from build123d import *

# Parameters (mm, degrees)
EXTRUDE_THIN1_DEPTH = 10
SKETCH2_W           = 17.824072676
SKETCH2_H           = 3.5
CUT_EXTRUDE1_DEPTH  = 10
SKETCH3_W           = 9
SKETCH3_H           = 3
BOSS_EXTRUDE1_DEPTH = 10
SKETCH4_R           = 1.75
CUT_EXTRUDE2_DEPTH  = 10
SKETCH5_W           = 15
SKETCH5_H           = 5.349927867
BOSS_EXTRUDE2_DEPTH = 27.0318
SKETCH6_W           = 9
SKETCH6_H           = 3.75
CUT_EXTRUDE3_DEPTH  = 13
BOSS_EXTRUDE3_DEPTH = 15
CUT_EXTRUDE8_REACH  = 67.42
SKETCH8_R           = 1.75
BOSS_EXTRUDE4_DEPTH = 37.0318
CUT_EXTRUDE6_DEPTH  = 11.169767789
SKETCH13_R          = 1.75
CUT_EXTRUDE9_DEPTH  = 3


with BuildPart() as part:
    # Sketch1 → Extrude-Thin1 (new body)
    with BuildSketch(Plane.XY):
        with BuildLine():
            Line((7.5, 8.014450411), (7.5, 13.364378278))
            Line((7.5, 13.364378278), (-7.5, 13.364378278))
            Line((-7.5, 13.364378278), (-7.5, 8.014450411))
            ThreePointArc((-7.5, 8.014450411), (0, -10.556649897), (7.5, 8.014450411))
        make_face()
        with BuildLine():
            Line((4.5, 6.614378278), (4.5, 10.364378278))
            Line((4.5, 10.364378278), (-4.5, 10.364378278))
            Line((-4.5, 10.364378278), (-4.5, 6.614378278))
            ThreePointArc((-4.5, 6.614378278), (0, -7.556649897), (4.5, 6.614378278))
        make_face(mode=Mode.SUBTRACT)
    extrude(amount=-EXTRUDE_THIN1_DEPTH)

    # Sketch2 → Cut-Extrude1 (cut)
    with BuildSketch(Plane(origin=(0, 0, -10), x_dir=(-1, 0, 0), z_dir=(0, 0, -1))):
        with Locations((8.912036338, 0)):
            Rectangle(SKETCH2_W, SKETCH2_H)
    extrude(amount=-CUT_EXTRUDE1_DEPTH, mode=Mode.SUBTRACT)

    # Sketch3 → Boss-Extrude1 (add)
    with BuildSketch(Plane.XY):
        with Locations((-12.153104343, 3.25)):
            Rectangle(SKETCH3_W, SKETCH3_H)
        with Locations((-12.04099167, -3.25)):
            Rectangle(SKETCH3_W, SKETCH3_H)
    extrude(amount=-BOSS_EXTRUDE1_DEPTH)

    # Sketch4 → Cut-Extrude2 (cut)
    with BuildSketch(Plane(origin=(0, 4.75, 0), x_dir=(1, 0, 0), z_dir=(0, 1, 0))):
        with Locations((-13.233947273, 5)):
            Circle(SKETCH4_R)
    extrude(amount=-CUT_EXTRUDE2_DEPTH, mode=Mode.SUBTRACT)

    # Sketch5 → Boss-Extrude2 (add)
    with BuildSketch(Plane.XY):
        with Locations((0, 10.689414345)):
            Rectangle(SKETCH5_W, SKETCH5_H)
    extrude(amount=BOSS_EXTRUDE2_DEPTH)

    # Sketch6 → Cut-Extrude3 (cut)
    with BuildSketch(Plane(origin=(0, 0, -10), x_dir=(-1, 0, 0), z_dir=(0, 0, -1))):
        with Locations((0, 8.489378278)):
            Rectangle(SKETCH6_W, SKETCH6_H)
    extrude(amount=-CUT_EXTRUDE3_DEPTH, mode=Mode.SUBTRACT)

    # Sketch7 → Boss-Extrude3 (add)
    with BuildSketch(Plane.ZY.offset(7.5)):
        Polygon((27.0318, 13.364378278), (-10, 13.364378278), (24.0318, 39.609893084), (24.0318, 51.294233998), (27.0318, 51.294233998), align=None)
    extrude(amount=-BOSS_EXTRUDE3_DEPTH)

    # Cut-Extrude8: up to this face of the body (flat: up to its plane)
    cut_extrude8_end = Plane(part.part.faces().sort_by_distance((0, 29.654342205, 27.0318))[0])
    # Sketch8 → Cut-Extrude8 (cut, up to the picked face)
    with BuildSketch(Plane(origin=(0, 0, -10), x_dir=(-1, 0, 0), z_dir=(0, 0, -1)), mode=Mode.PRIVATE) as cut_extrude8_sk1:
        with Locations(Location((0.697367247, 45.709350103, 0), (0, 0, 90))):
            Circle(SKETCH8_R)
    cut_extrude8_tool1 = split(extrude(cut_extrude8_sk1.sketch, amount=-CUT_EXTRUDE8_REACH, mode=Mode.PRIVATE), bisect_by=cut_extrude8_end, keep=Keep.BOTH, mode=Mode.PRIVATE)
    # Sketch8 → Cut-Extrude8 (cut, up to the picked face)
    with BuildSketch(Plane(origin=(0, 0, -10), x_dir=(-1, 0, 0), z_dir=(0, 0, -1)), mode=Mode.PRIVATE) as cut_extrude8_sk2:
        Polygon((6.282251141, 44.365676022), (6.282251141, 47.053024185), (6.282251141, 51.294233998), (7.5, 51.294233998), (7.5, 39.609893084), (7.5, 13.364378278), align=None)
    cut_extrude8_tool2 = split(extrude(cut_extrude8_sk2.sketch, amount=-CUT_EXTRUDE8_REACH, mode=Mode.PRIVATE), bisect_by=cut_extrude8_end, keep=Keep.BOTH, mode=Mode.PRIVATE)
    # Sketch8 → Cut-Extrude8 (cut, up to the picked face)
    with BuildSketch(Plane(origin=(0, 0, -10), x_dir=(-1, 0, 0), z_dir=(0, 0, -1)), mode=Mode.PRIVATE) as cut_extrude8_sk3:
        Polygon((-4.887516648, 47.053024185), (-4.887516648, 44.365676022), (-7.5, 13.364378278), (-7.5, 39.609893084), (-7.5, 51.294233998), (-4.887516648, 51.294233998), align=None)
    cut_extrude8_tool3 = split(extrude(cut_extrude8_sk3.sketch, amount=-CUT_EXTRUDE8_REACH, mode=Mode.PRIVATE), bisect_by=cut_extrude8_end, keep=Keep.BOTH, mode=Mode.PRIVATE)
    add(cut_extrude8_tool1.solids().sort_by(Axis((-0.697367, 45.70935, -10), (0, 0, 1)))[0], mode=Mode.SUBTRACT)
    add(cut_extrude8_tool2.solids().sort_by(Axis((-7.031388, 38.294234, -10), (0, 0, 1)))[0], mode=Mode.SUBTRACT)
    add(cut_extrude8_tool3.solids().sort_by(Axis((6.494669, 38.294234, -10), (0, 0, 1)))[0], mode=Mode.SUBTRACT)

    # Sketch11 → Boss-Extrude4 (add)
    with BuildSketch(Plane(origin=(0, 0, -10), x_dir=(-1, 0, 0), z_dir=(0, 0, -1))):
        with BuildLine():
            Line((6.282251141, -43.878975815), (6.282251141, -46.566323978))
            Line((6.282251141, -46.566323978), (6.282251141, -50.807533791))
            Line((6.282251141, -50.807533791), (2.041041328, -50.807533791))
            Line((2.041041328, -50.807533791), (-0.646306835, -50.807533791))
            Line((-0.646306835, -50.807533791), (-4.887516648, -50.807533791))
            Line((-4.887516648, -50.807533791), (-4.887516648, -46.566323978))
            Line((-4.887516648, -46.566323978), (-4.887516648, -43.878975815))
            Line((-4.887516648, -43.878975815), (-4.887516648, -5.83548046))
            ThreePointArc((-4.887516648, -5.83548046), (1.037871953, -7.540787293), (6.282251141, -4.298135849))
            Line((6.282251141, -4.298135849), (6.282251141, -43.878975815))
        make_face()
    extrude(amount=-BOSS_EXTRUDE4_DEPTH)

    # Sketch12 → Cut-Extrude6 (cut)
    with BuildSketch(Plane(origin=(-6.282251141, 0, 0), x_dir=(0, 0, -1), z_dir=(1, 0, 0))):
        Polygon((10, -12.309364669), (10, -50.807533791), (-24.0318, -50.807533791), (-24.0318, -39.062586463), align=None)
    extrude(amount=CUT_EXTRUDE6_DEPTH, mode=Mode.SUBTRACT)

    # Sketch13 → Cut-Extrude9 (cut)
    with BuildSketch(Plane.XY.offset(27.0318)):
        with Locations((-0.697367247, -45.222649897)):
            Circle(SKETCH13_R)
    extrude(amount=-CUT_EXTRUDE9_DEPTH, mode=Mode.SUBTRACT)


solid = part.part
Here's how the part is built. I have some questions about the finished solid (model axes, mm). A direction names the side the tool comes from. Coordinates: 2 decimals unless noted, no trailing zeros. Order: outer loops, then holes, each group sorted by start corner. A loop starts at its lowest first (then second) coordinate and runs counter-clockwise, first axis right, second up. Notation, with made-up numbers: M 5,22.5 L 40,22.5 A19 ccw 40,32.5 Z; hole C 84.5,32.5 d2. An arc over 180 degrees is marked long. Answer as CSV lines item,"result".
Item 1: Imagine slicing it at B-B on x = -13.75. Write out the boundary of the cut face in (y, z).
Results found:
outline,"M -4.75,-10 L -1.75,-10 L -1.75,-6.67 L -4.75,-6.67 Z; M -4.75,-3.33 L -1.75,-3.33 L -1.75,0 L -4.75,0 Z; M 1.75,-10 L 4.75,-10 L 4.75,-6.67 L 1.75,-6.67 Z; M 1.75,-3.33 L 4.75,-3.33 L 4.75,0 L 1.75,0 Z"
Item 2: Imagine slicing it at A-A on z = 2. Write out the boundary of the cut face in (x, y), plus the area to 3 significant figures.
Results found:
outline,"M -7.5,8.01 L -4.5,8.01 L -4.5,10.36 L 4.5,10.36 L 4.5,8.01 L 7.5,8.01 L 7.5,13.36 L 6.72,22.62 L -7.14,22.62 L -7.5,13.36 Z; M -6.28,-21.74 L 4.89,-21.74 L 4.89,-5.84 A7.61 cw -6.28,-4.3 Z"
area,"359 mm2"
Item 3: If I drill on line 1 (X direction, y = 8, z = -1.5); line 2 (X direction, y = 4, z = -5); line 3 (X direction, y = -3.4, z = -5), over which ranges is the centre line in solid material (lowest first)?
Results found:
line 1,"-7.51 to -4.5, 4.5 to 7.51"
line 2,"-16.65 to -14.98, -11.48 to -6.84, 6.84 to 10.13"
line 3,"-16.54 to -14.98, -11.48 to -6.9, 6.9 to 10.17"
Item 4: We'd pull the mould along X, two halves only. Please class faces 6 (the face through (4.888, 48, 26)), 7 (the face through (-11, 1.75, -5)), 8 (the face through (-6.523, 4.521, -4.93)), 9 (the face through (-7.5, 11, 9)): +X half, -X half, draft (parallel to the pull), parting line (faces both ways), or undercut.
Results found:
face 6,"+X half"
face 7,"draft"
face 8,"undercut"
face 9,"-X half"
Item 5: Imagine slicing it at D-D on z = -5. Give the number of separate pieces and of enclosed holes in the cut face, plus the area to 3 significant figures.
Results found:
separate pieces,"3"
enclosed holes,"0"
area,"332 mm2"
Item 6: Imagine slicing it at C-C on x = 6.5. Write out the boundary of the cut face in (y, z).
Results found:
outline,"M -8.38,-10 L -4.07,-10 L -4.07,0 L -8.38,0 Z; M 4.55,-10 L 13.36,-10 L 25.23,5.39 L 25.23,27.03 L 8.01,27.03 L 8.01,0 L 4.55,0 Z"
Item 7: For pin 1 (2 mm diameter, centred on x = -2, z = 3, fed in from +Y); pin 2 (4 mm diameter, centred on x = -13.23, z = -5, fed in from -Y); pin 3 (2 mm diameter, centred on x = -1.5, y = -6.5, fed in from +Z); pin 4 (2.5 mm diameter, centred on y = 48.5, z = 25, fed in from -X), each with a flat end and sliding along its axis, tell me the tip position at first contact or that it passes through.
Results found:
pin 1,"y = 24.16"
pin 2,"y = -4.75"
pin 3,"z = 27.03"
pin 4,"x = -6.28"
Item 8: On a 3-axis mill with a long thin cutter (end or side, diameter ignored), from which of +Z, -Z, +X, -X, +Y, -Y can I reach the whole of each face in a straight line? I mean faces 1 (the face through (-7.044, -3.106, -4.93)), 2 (the face through (-15, -4.75, -4)), 3 (the face through (0, 8.014, 13)), 4 (the face through (-2, 44, 24.032)), 5 (the face through (-2, -43.7, 24.032)). Say none if no direction works.
Results found:
face 1,"+Z, -Z"
face 2,"+Z, -Z, -X, -Y"
face 3,"+Z, +X, -X"
face 4,"-Z, +X, -X, +Y"
face 5,"-Z, +X, -X, -Y"
